```python
from build123d import *

# Parameters (mm, degrees)
SKETCH_1_R          = 6
EXTRUDE_1_DEPTH     = 10
SKETCH_3_W          = 5
SKETCH_3_H          = 8
EXTRUDE_2_DEPTH     = 50
SKETCH_2_R          = 3
CUT_EXTRUDE_1_DEPTH = 30
SKETCH_14_W         = 15
SKETCH_14_H         = 18
EXTRUDE_7_DEPTH     = 5
FILLET_2_R          = 5
FILLET_3_R          = 10
SKETCH_15_R         = 2
CUT_EXTRUDE_4_DEPTH = 5


with BuildPart() as part:
    # 草图1 → 凸台-拉伸1 (new body)
    with BuildSketch(Plane.XY):
        Circle(SKETCH_1_R)
    extrude(amount=EXTRUDE_1_DEPTH)

    # 草图3 → 凸台-拉伸2 (add)
    with BuildSketch(Plane(origin=(0, 0, 0), x_dir=(0, 0, -1), z_dir=(1, 0, 0))):
        with Locations((-2.5, 0)):
            Rectangle(SKETCH_3_W, SKETCH_3_H)
    extrude(amount=EXTRUDE_2_DEPTH)

    # 草图2 → 切除-拉伸1 (cut)
    with BuildSketch(Plane.XY.offset(10)):
        Circle(SKETCH_2_R)
    extrude(amount=-CUT_EXTRUDE_1_DEPTH, mode=Mode.SUBTRACT)

    # 镜向1: part across plane


with BuildPart() as part_1:
    add(part.part)
    add(part.part.mirror(Plane.ZY.offset(-50)))

    # 草图14 → 凸台-拉伸7 (add)
    with BuildSketch(Plane(origin=(0, 0, 0), x_dir=(-1, 0, 0), z_dir=(0, 0, -1))):
        with Locations((-50, 13)):
            Rectangle(SKETCH_14_W, SKETCH_14_H)
    extrude(amount=-EXTRUDE_7_DEPTH)

    # 圆角2
    fillet_2_edges = [part_1.edges().sort_by_distance(p)[0] for p in [
        (57.5, 22, 2.5),
        (42.5, 22, 2.5),
    ]]
    fillet(fillet_2_edges, radius=FILLET_2_R)

    # 圆角3
    fillet_3_edges = [part_1.edges().sort_by_distance(p)[0] for p in [
        (42.5, 4, 2.5),
        (57.5, 4, 2.5),
    ]]
    fillet(fillet_3_edges, radius=FILLET_3_R)

    # 草图15 → 切除-拉伸4 (cut)
    with BuildSketch(Plane(origin=(0, 0, 0), x_dir=(-1, 0, 0), z_dir=(0, 0, -1))):
        with Locations((-50, 16.57)):
            Circle(SKETCH_15_R)
    extrude(amount=-CUT_EXTRUDE_4_DEPTH, mode=Mode.SUBTRACT)


solid = part_1.part
```
For this review, take the finished solid that the model builds, in its own axes (mm). A direction names the side the tool comes from. Coordinates: 2 decimals unless noted, no trailing zeros. Loops run counter-clockwise (first coordinate to the right, second up) from the corner with the lowest first, then second, coordinate; pieces in that order, holes last. Notation, with made-up numbers: (23, 56.25) - (37, 56.25) arc R9 cw to (37, 68.25) - close; hole circle Ø11 at (23.5, 52.5). An arc over 180 degrees is marked (long way). Use one line per item in the form item = value. Start each with the question number.
1) To check wall thickness, follow probe 1 along Y at (x, z) = (100, 6.5); probe 2 along Y at (x, z) = (9.5, 2); probe 3 along X at (y, z) = (-1.5, 7.25). State the ranges of each line that lie inside material, in increasing order. Write a range as from..to.
2) Draft analysis for pull direction Y (two halves, no side actions). For faces 4 (the face through (-3, 0, 5)), 5 (the face through (106, 0, 5)), 6 (the face through (50, 2, 0)), state which applies: released by +Y, released by -Y, zero draft, split by the parting line, or undercut.
3) For pin 1 (10 mm diameter, centred on x = 30, y = 3.5, fed in from +Z); pin 2 (1.5 mm diameter, centred on x = 30, z = 4, fed in from -Y); pin 3 (3 mm diameter, centred on x = 85.5, z = 1.5, fed in from +Y), all flat-tipped, find the tip position at first contact; note any pin that passes through.
4) Take a section at C-C (z = 2.25). State the section outline as (x, y) points.
5) Take a section at D-D (z = 6.75). State the section outline as (x, y) points, plus the area to 3 significant figures.
6) Take a section at B-B (y = 0). State the section outline as (x, z) points.
7) For faces 1 (the face through (57.5, 15, 2)), 2 (the face through (42.5, 15, 2)), 3 (the face through (51, -4, 3)), list the 3-axis set-ups (+Z, -Z, +X, -X, +Y, -Y) from which the entire face can be reached by the end or side of a thin tool; tool diameter is ignored.
8) Take a section at A-A (x = 50). State the section outline as (y, z) points.
From the geometry:
q1.probe_1 = -6..-3, 3..6
q1.probe_2 = -4..4
q1.probe_3 = -5.81..-2.6, 2.6..5.81, 94.19..97.4, 102.6..105.81
q2.face_4 = undercut
q2.face_5 = split by the parting line
q2.face_6 = zero draft
q3.pin_1 = 5
q3.pin_2 = -4
q3.pin_3 = 4
q4.outline = (4.47, -4) - (95.53, -4) arc R6 ccw (long way) to (95.53, 4) - (67.5, 4) arc R10 cw to (57.5, 14) - (57.5, 17) arc R5 ccw to (52.5, 22) - (47.5, 22) arc R5 ccw to (42.5, 17) - (42.5, 14) arc R10 cw to (32.5, 4) - (4.47, 4) arc R6 ccw (long way) to start; hole circle Ø6 at (0, 0); hole circle Ø4 at (50, 16.57); hole circle Ø6 at (100, 0)
q5.outline = circle Ø12 at (0, 0); circle Ø12 at (100, 0); hole circle Ø6 at (0, 0); hole circle Ø6 at (100, 0)
q5.area = 170 mm2
q6.outline = (-6, 0) - (-3, 0) - (-3, 10) - (-6, 10) - close; (3, 0) - (97, 0) - (97, 10) - (94, 10) - (94, 5) - (6, 5) - (6, 10) - (3, 10) - close; (103, 0) - (106, 0) - (106, 10) - (103, 10) - close
q7.face_1 = +Z, -Z, +X, +Y
q7.face_2 = +Z, -Z, -X, +Y
q7.face_3 = +Z, -Z, -Y
q8.outline = (-4, 0) - (14.57, 0) - (14.57, 5) - (-4, 5) - close; (18.57, 0) - (22, 0) - (22, 5) - (18.57, 5) - close
